Could you check a few things on this model? Use its own coordinates, in mm. A direction names the side the tool comes from. Coordinates: 2 decimals unless noted, no trailing zeros. Write each loop counter-clockwise with the first axis right and the second up, starting at its lowest first coordinate (ties: lowest second). Pieces come first, ordered by that corner, then holes.
Item 1: Thinking about a two-plate mould opening in Z: for faces 5 (the flat face through (5, 1, 0)), 6 (the flat face through (5, 1, -20)), 7 (the flat face through (14.5, 1, -5)), 8 (the flat face through (0.5, 1, -10)), which applies, +Z half, -Z half, draft (parallel to the pull), parting line (faces both ways), or undercut?
Item 2: I want a section at A-A on z = -10. Please give me the cut outline in (x, y).
Item 3: I want a section at B-B on x = 5. Please give me the cut outline in (y, z).
Item 4: I want a section at D-D on x = -2.25. Please give me the cut outline in (y, z), then the cut area to 3 significant figures.
Item 5: I want a section at C-C on y = 0.6. Please give me the cut outline in (x, z).
Item 6: If I drill on probe 1 along Z at (x, y) = (5, 1.65); probe 2 along X at (y, z) = (2.5, -6.5); probe 3 along X at (y, z) = (1, -9.25), over which ranges is the centre line in solid material (lowest first)?
Item 7: For P1, Ø1.5, axis at x = -3, y = 2, coming from the +Z side; P2, Ø1.5, axis at x = 16.5, y = 1, coming from the -Z side; P3, Ø1.5, axis at x = 15.5, y = 2, coming from the +Z side, each with a flat end and sliding along its axis, tell me the tip position at first contact or that it passes through.
Item 8: Which directions (+Z, -Z, +X, -X, +Y, -Y) give clear straight access to the entire face, cutting with the end or side of a thin tool? Please do faces 1 (the flat face through (10, 1, -2)), 2 (the flat face through (0, 1, -2)), 3 (the flat face through (12, 1, -17)), 4 (the flat face through (0, 1, -18)).
Autodesk Inventor part; units mm, degrees
ref_plane "YZ Plane" through (0, 0, 0) normal (1, 0, 0) x (0, 1, 0)
ref_plane "XZ Plane" through (0, 0, 0) normal (0, 1, 0) x (-1, 0, 0)
ref_plane "XY Plane" through (0, 0, 0) normal (0, 0, 1) x (1, 0, 0)
sketch "Boceto1" plane through (0, 0, 0) normal (0, 1, 0) x (-1, 0, 0)
  line L0 (0, 0) -> (-10, 0)
  line L1 (-17.5, -7.5) -> (-17.5, -12.5)
  line L2 (-10, -20) -> (0, -20)
  line L3 (5.5, -17) -> (5.5, -3)
  line L4 (0, -3) -> (0, 0)
  line L5 (-10, -3) -> (-10, 0)
  line L6 (-14.5, -3) -> (-10, -3)
  line L7 (0, -3) -> (5.5, -3)
  line L8 (0, -17) -> (0, -20)
  line L9 (-10, -17) -> (-10, -20)
  line L10 (5.5, -17) -> (0, -17)
  line L11 (-10, -17) -> (-14.5, -17)
  line L12 (-14.5, -12.5) -> (-17.5, -12.5)
  line L13 (-14.5, -7.5) -> (-17.5, -7.5)
  line L14 (-14.5, -17) -> (-14.5, -12.5)
  line L15 (-14.5, -7.5) -> (-14.5, -3)
  circle A0 centre (-5, -10) radius 2.5
  line L16 (-0.5, -8) -> (-0.5, -12)
  line L17 (-0.5, -12) -> (3.5, -12)
  line L18 (3.5, -12) -> (3.5, -8)
  line L19 (3.5, -8) -> (-0.5, -8)
  point P0 (-17.5, -10)
  point P1 (-5, -20)
  point P2 (-0.5, -10)
  dimension "d0" = 23
  dimension "d1" = 20
  dimension "d4" = 10
  dimension "d6" = 5
  dimension "d7" = 3
  dimension "d8" = 3
  dimension "d10" = 5
  dimension "d13" = 7.5
  dimension "d14" = 4
  dimension "d15" = 4
  dimension "d16" = 2
extrude "Extrusión2" add sketch "Boceto1" along normal blind 3
properties part number "Barilla" material "Oro"
Response values:
1. face 5: +Z half
1. face 6: -Z half
1. face 7: draft
1. face 8: undercut
2. outline: (-5.5, 0) - (-3.5, 0) - (-3.5, 3) - (-5.5, 3) - close; (0.5, 0) - (2.5, 0) - (2.5, 3) - (0.5, 3) - close; (7.5, 0) - (17.5, 0) - (17.5, 3) - (7.5, 3) - close
3. outline: (0, -20) - (3, -20) - (3, -12.5) - (0, -12.5) - close; (0, -7.5) - (3, -7.5) - (3, 0) - (0, 0) - close
4. outline: (0, -17) - (3, -17) - (3, -12) - (0, -12) - close; (0, -8) - (3, -8) - (3, -3) - (0, -3) - close
4. area: 30.0 mm2
5. outline: (-5.5, -17) - (0, -17) - (0, -20) - (10, -20) - (10, -17) - (14.5, -17) - (14.5, -12.5) - (17.5, -12.5) - (17.5, -7.5) - (14.5, -7.5) - (14.5, -3) - (10, -3) - (10, 0) - (0, 0) - (0, -3) - (-5.5, -3) - close; hole (-3.5, -12) - (0.5, -12) - (0.5, -8) - (-3.5, -8) - close; hole circle Ø5 at (5, -10)
6. probe 1: z = -20 to -12.5, -7.5 to 0
6. probe 2: x = -5.5 to 14.5
6. probe 3: x = -5.5 to -3.5, 0.5 to 2.62, 7.38 to 17.5
7. P1: stops at z = -3
7. P2: stops at z = -12.5
7. P3: stops at z = -7.5
8. face 1: +Z, +X, +Y, -Y
8. face 2: +Z, -X, +Y, -Y
8. face 3: -Z, +X, +Y, -Y
8. face 4: -Z, -X, +Y, -Y
